Here's the drawing with two shaded views (mm, measured from the low corner). I have some questions. Give positions to 0.01 mm unless a question says otherwise; leave off trailing zeros. Write each loop counter-clockwise with the first axis right and the second up, starting at its lowest first coordinate (ties: lowest second). Pieces come first, ordered by that corner, then holes. Notation, with made-up numbers: (59.25, 77) - (118.25, 77) arc R30 ccw to (118.25, 113) - close; hole circle Ø6 at (12.25, 63). An arc over 180 degrees is marked (long way). Answer as a JSON object with one key per item and string values. Group by question number.
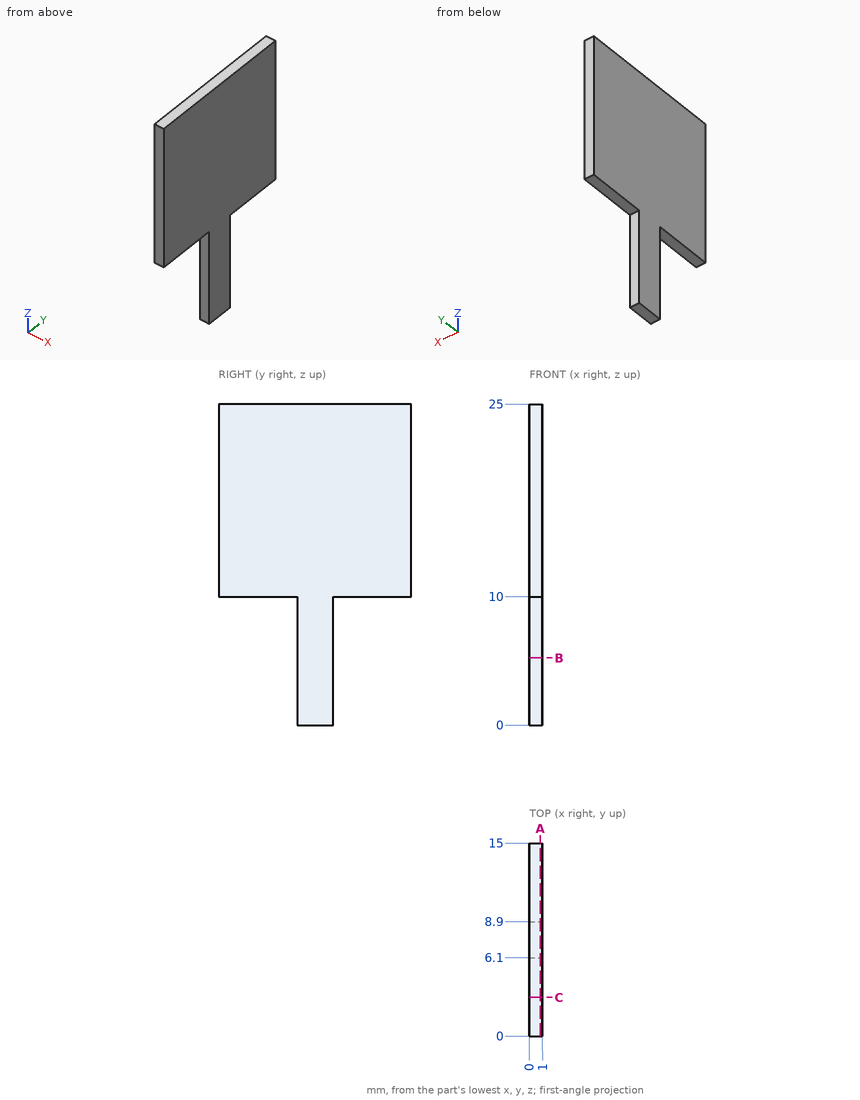
(1) I need wall thicknesses on L1, parallel to Z at x = 0.75, y = 13.5; L2, parallel to Y at x = 0.35, z = 8.75. Which ranges of each line are inside material? Lowest first, please.
(2) I want a section at C-C, the plane y = 3. Please give me the cut outline in (x, z).
(3) I want a section at A-A, the plane x = 0.85. Please give me the cut outline in (y, z), and give its area (3 significant figures).
(4) Will this pin go through, and if not, where does the flat tip stop? P1, Ø5, axis at y = 8, z = 10.5, coming from the -X side.
(5) I want a section at B-B, the plane z = 5.25. Please give me the cut outline in (x, y).
Entries:
{
 "1": {"L1": "10 to 25", "L2": "6.1 to 8.9"},
 "2": {"outline": "(0, 10) - (1, 10) - (1, 25) - (0, 25) - close"},
 "3": {"outline": "(0, 10) - (6.1, 10) - (6.1, 0) - (8.9, 0) - (8.9, 10) - (15, 10) - (15, 25) - (0, 25) - close", "area": "253 mm^2"},
 "4": {"P1": "x = 0"},
 "5": {"outline": "(0, 6.1) - (1, 6.1) - (1, 8.9) - (0, 8.9) - close"}
}
